Work out the finished part from the listing and answer in its coordinate system (mm). A direction names the side the tool comes from. Coordinates: 2 decimals unless noted, no trailing zeros. Order: outer loops, then holes, each group sorted by start corner. A loop starts at its lowest first (then second) coordinate and runs counter-clockwise, first axis right, second up. Notation, with made-up numbers: M 30,9.25 L 59,9.25 A10 cw 59,27.25 Z; hole C 11.5,43.5 d3. An arc over 180 degrees is marked long. Use a Markdown table: item, result.
from build123d import *

# Parameters (mm, degrees)
CROQUIS1_R              = 6.45
CROQUIS1_R_2            = 6.5
SALIENTE_EXTRUIR1_DEPTH = 35
CROQUIS2_R              = 2
CORTAR_EXTRUIR1_DEPTH   = 10


with BuildPart() as part:
    # Croquis1 → Saliente-Extruir1 (new body)
    with BuildSketch(Plane.XY):
        with BuildLine():
            Line((10, 28), (10, 0))
            ThreePointArc((10, 0), (0, -10), (-10, 0))
            Line((-10, 0), (-10, 28))
            ThreePointArc((-10, 28), (0, 38), (10, 28))
        make_face()
        Circle(CROQUIS1_R, mode=Mode.SUBTRACT)
        with Locations((0, 28)):
            Circle(CROQUIS1_R_2, mode=Mode.SUBTRACT)
    extrude(amount=SALIENTE_EXTRUIR1_DEPTH)

    # Croquis2 → Cortar-Extruir1 (cut)
    with BuildSketch(Plane(origin=(0, 0, 0), x_dir=(1, 0, 0), z_dir=(0, 1, 0))):
        with Locations(Location((0, -7.5, 0), (0, 0, 270))):
            Circle(CROQUIS2_R)
        with Locations(Location((0, -27.5, 0), (0, 0, 270))):
            Circle(CROQUIS2_R)
    extrude(amount=-CORTAR_EXTRUIR1_DEPTH, mode=Mode.SUBTRACT)


solid = part.part
(1) Straight lines are drawn through the part: L1, parallel to Z at x = 0, y = -7.7; L2, parallel to Y at x = -3.5, z = 11.5; L3, parallel to Y at x = -2.5, z = 27.5. For each, find the intervals that lie inside material, in ascending order.
Conclusion:
| item | result |
|---|---|
| L1 | 0 to 5.5, 9.5 to 25.5, 29.5 to 35 |
| L2 | -9.37 to -5.42, 5.42 to 22.52, 33.48 to 37.37 |
| L3 | -9.68 to -5.95, 5.95 to 22, 34 to 37.68 |
(2) A cutting plane is placed at C-C (x = 5). Determine the outline of the cut face in (y, z).
Conclusion:
| item | result |
|---|---|
| outline | M -8.66,0 L -4.07,0 L -4.07,35 L -8.66,35 Z; M 4.07,0 L 23.85,0 L 23.85,35 L 4.07,35 Z; M 32.15,0 L 36.66,0 L 36.66,35 L 32.15,35 Z |
(3) A cutting plane is placed at B-B (z = 22). Determine the outline of the cut face in (x, y), then the cut area to 3 significant figures.
Conclusion:
| item | result |
|---|---|
| outline | M -10,0 A10 ccw 10,0 L 10,28 A10 ccw -10,28 Z; hole C 0,28 d13; hole C 0,0 d12.9 |
| area | 611 mm2 |
(4) A cutting plane is placed at A-A (x = 0). Determine the outline of the cut face in (y, z).
Conclusion:
| item | result |
|---|---|
| outline | M -10,0 L -6.45,0 L -6.45,5.5 L -10,5.5 Z; M -10,9.5 L -6.45,9.5 L -6.45,25.5 L -10,25.5 Z; M -10,29.5 L -6.45,29.5 L -6.45,35 L -10,35 Z; M 6.45,0 L 21.5,0 L 21.5,35 L 6.45,35 Z; M 34.5,0 L 38,0 L 38,35 L 34.5,35 Z |
(5) A cutting plane is placed at D-D (z = 27.5). Determine the outline of the cut face in (x, y), then the cut area to 3 significant figures.
Conclusion:
| item | result |
|---|---|
| outline | M -10,0 A10 ccw -2,-9.8 L -2,-6.13 A6.45 cw long 2,-6.13 L 2,-9.8 A10 ccw 10,0 L 10,28 A10 ccw -10,28 Z; hole C 0,28 d13 |
| area | 596 mm2 |
(6) Determine the mould class of faces 3 (the cylindrical face through (-0.846, 34.445, 17.255)), 4 (the cylindrical face through (0, 38, 17)), 5 (the flat face through (10, 14, 17)) for opening direction Y: pulls with the +Y half, pulls with the -Y half, needs draft (parallel to the pull), parting line crosses it, or undercut.
Conclusion:
| item | result |
|---|---|
| face 3 | undercut |
| face 4 | pulls with the +Y half |
| face 5 | needs draft |
(7) Which of the six approach directions +Z, -Z, +X, -X, +Y, -Y give full straight-line access (tool end or side, diameter ignored) to faces 1 (the cylindrical face through (1.983, -8.039, 7.24)), 2 (the cylindrical face through (0, -10, 17))?
Conclusion:
| item | result |
|---|---|
| face 1 | -Y |
| face 2 | +Z, -Z, -Y |
(8) Given P1, Ø3.5, axis at x = 0, z = 27.5, coming from the -Y side; P2, Ø1.5, axis at x = -8, z = 9, coming from the +Y side; P3, Ø3, axis at y = -3.5, z = 24, coming from the +X side; P4, Ø11.5, axis at x = 0, y = 0, coming from the -Z side (1 decimal), each flat-ended and moving along its own axis, determine where each tip first touches the part or whether it passes through.
Conclusion:
| item | result |
|---|---|
| P1 | y = 6.21 |
| P2 | y = 34.89 |
| P3 | x = 9.8 |
| P4 | through |
